from build123d import *

# Parameters (mm, degrees)
CHAMFER2_SIZE           = 1.778
CHAMFER2_SIZE2          = 2.54
SKETCH2_W               = 4.064
SKETCH2_H               = 3.048
CUT_EXTRUDE1_DEPTH      = 9.382
CUT_EXTRUDE1_DEPTH_BACK = 9.382
CUT_EXTRUDE2_DEPTH      = 9.382
CUT_EXTRUDE2_DEPTH_BACK = 9.382


with BuildPart() as part:
    # Sketch1 → Base-Revolve (revolve)
    with BuildSketch(Plane.XY):
        Polygon((3.556, 73.406), (3.556, 0), (6.35, 0), (8.382, 3.048), (8.382, 5.588), (5.969, 5.588), (5.969, 73.406), align=None)
    revolve(axis=Axis((0, 0, 0), (0, 1, 0)))

    # Chamfer2
    chamfer2_edges = [part.edges().sort_by_distance(p)[0] for p in [
        (-3.556, 0, 0),
    ]]
    chamfer2_side = [part.faces().sort_by_distance(p)[0] for p in [
        (-3.735605122, 0, 0),
    ]]
    chamfer(chamfer2_edges, length=CHAMFER2_SIZE, length2=CHAMFER2_SIZE2, reference=chamfer2_side[0])

    # Sketch2 → Cut-Extrude1 (cut, two sides)
    with BuildSketch(Plane.XY) as cut_extrude1_sk:
        with Locations((0, 1.524)):
            Rectangle(SKETCH2_W, SKETCH2_H)
    extrude(amount=CUT_EXTRUDE1_DEPTH, mode=Mode.SUBTRACT)
    extrude(cut_extrude1_sk.sketch, amount=-CUT_EXTRUDE1_DEPTH_BACK, mode=Mode.SUBTRACT)

    # Sketch3 → Cut-Extrude2 (cut, two sides)
    with BuildSketch(Plane.XY) as cut_extrude2_sk:
        Polygon((-7.874, 5.08), (-7.874, 2.286), (-8.382, 3.048), (-8.382, 5.08), align=None)
    extrude(amount=CUT_EXTRUDE2_DEPTH, mode=Mode.SUBTRACT)
    extrude(cut_extrude2_sk.sketch, amount=-CUT_EXTRUDE2_DEPTH_BACK, mode=Mode.SUBTRACT)


solid = part.part
Model file for the job. Use its own axes, mm. A direction names the side the tool comes from. Round coordinates to 2 decimals unless told otherwise and drop trailing zeros. Order: outer loops, then holes, each group sorted by start corner. A loop starts at its lowest first (then second) coordinate and runs counter-clockwise, first axis right, second up. Notation, with made-up numbers: M 0.5,42.5 L 5.5,42.5 A29 ccw 5.5,69.5 Z; hole C 10.5,61.5 d11. An arc over 180 degrees is marked long. Write each question's results on one line, items separated by ' | '. Start each with the question number.
(1) Probe probe 1 along Z at (x, y) = (0, 52); probe 2 along Z at (x, y) = (0.25, 64.5). List the from-to ranges inside material, lowest first. Write a range as from..to.
(2) Saw through at A-A, the plane z = 0. Give the cut face in (x, y), then the cut area to 3 significant figures.
(3) Drop flat-ended pins along their axis: pin 1 (6.5 mm diameter, centred on x = 0, z = 0, fed in from -Y); pin 2 (4.5 mm diameter, centred on x = -0.5, z = 5.5, fed in from -Y); pin 3 (0.9 mm diameter, centred on y = 1.5, z = 4.5, fed in from +X); pin 4 (3.5 mm diameter, centred on y = 1.5, z = -6.5, fed in from -X). Give the stop position or say it passes through.
(4) Which spindle directions (+Z, -Z, +X, -X, +Y, -Y) get a long thin tool onto all of the face, cutting with end or side? Do faces 5 (the face through (2.032, 2, -5)), 6 (the face through (-1.294, 39.972, 5.827)), 7 (the face through (-5.5, 0, 0)). Say none if no direction does.
(5) Saw through at C-C, the plane y = 43.5. Give the cut face in (x, z), then the cut area to 3 significant figures.
(6) Saw through at B-B, the plane x = 0. Give the cut face in (y, z), then the cut area to 3 significant figures.
(7) Two-plate mould, pull along Z, no slides. Class faces 1 (the face through (-4.234, 1.57, -0.07)), 2 (the face through (6.7, 0.53, 0.12)), 3 (the face through (4.234, 1.57, 0.07)), 4 (the face through (-7.874, 4, 0)): pulls with the +Z half, pulls with the -Z half, needs draft (parallel to the pull), parting line crosses it, or undercut.
Established:
1) probe 1: z = -5.97..-3.56, 3.56..5.97 | probe 2: z = -5.96..-3.55, 3.55..5.96
2) outline: M -8.38,5.08 L -7.87,5.08 L -7.87,2.29 L -6.35,0 L -5.33,0 L -3.56,2.54 L -3.56,73.41 L -5.97,73.41 L -5.97,5.59 L -8.38,5.59 Z; M 3.56,2.54 L 5.33,0 L 6.35,0 L 8.38,3.05 L 8.38,5.59 L 5.97,5.59 L 5.97,73.41 L 3.56,73.41 Z | area: 369 mm^2
3) pin 1: passes through | pin 2: stops at y = 0 | pin 3: stops at x = 6.3 | pin 4: stops at x = -6.26
4) face 5: +Z, -Z, -Y | face 6: +Y | face 7: +Z, -Z, +X, -X, -Y
5) outline: C 0,0 d11.94; hole C 0,0 d7.11 | area: 72.2 mm^2
6) outline: M 3.05,-8.38 L 5.59,-8.38 L 5.59,-5.97 L 73.41,-5.97 L 73.41,-3.56 L 3.05,-3.56 Z; M 3.05,3.56 L 73.41,3.56 L 73.41,5.97 L 5.59,5.97 L 5.59,8.38 L 3.05,8.38 Z | area: 352 mm^2
7) face 1: undercut | face 2: parting line crosses it | face 3: undercut | face 4: needs draft
